Source: CAD feature listing. Evaluate the final solid. Frame: model axes, mm. Face numbers are marked on the shaded views. A direction names the side the tool comes from. Give positions to 0.01 mm unless a question says otherwise; leave off trailing zeros. Write each loop counter-clockwise with the first axis right and the second up, starting at its lowest first coordinate (ties: lowest second). Pieces come first, ordered by that corner, then holes.
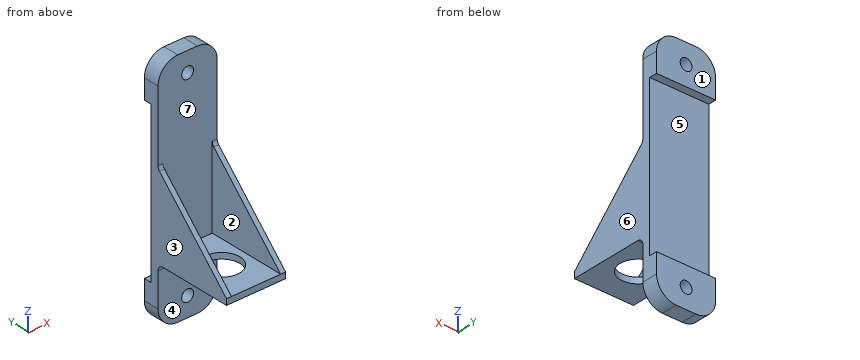
```python
from build123d import *

# Parameters (mm, degrees)
SKETCH1_W           = 30
SKETCH1_H           = 120
BOSS_EXTRUDE1_DEPTH = 8
SKETCH2_W           = 30
SKETCH2_H           = 80
CUT_EXTRUDE1_DEPTH  = 4
SKETCH3_W           = 30
SKETCH3_H           = 3
BOSS_EXTRUDE2_DEPTH = 40
SKETCH4_R           = 9.1
CUT_EXTRUDE2_DEPTH  = 40
BOSS_EXTRUDE3_DEPTH = 2.5
BOSS_EXTRUDE4_DEPTH = 2.5
SKETCH7_R           = 3
CUT_EXTRUDE3_DEPTH  = 131
FILLET1_R           = 10
FILLET2_R           = 3
FILLET3_R           = 3


with BuildPart() as part:
    # Sketch1 → Boss-Extrude1 (new body)
    with BuildSketch(Plane(origin=(0, 0, 0), x_dir=(1, 0, 0), z_dir=(0, 1, 0))):
        with Locations((15, 60)):
            Rectangle(SKETCH1_W, SKETCH1_H)
    extrude(amount=BOSS_EXTRUDE1_DEPTH)

    # Sketch2 → Cut-Extrude1 (cut)
    with BuildSketch(Plane(origin=(0, 8, 0), x_dir=(1, 0, 0), z_dir=(0, 1, 0))):
        with Locations((15, 60)):
            Rectangle(SKETCH2_W, SKETCH2_H)
    extrude(amount=-CUT_EXTRUDE1_DEPTH, mode=Mode.SUBTRACT)

    # Sketch3 → Boss-Extrude2 (add)
    with BuildSketch(Plane.XZ):
        with Locations((15, -88.5)):
            Rectangle(SKETCH3_W, SKETCH3_H)
    extrude(amount=BOSS_EXTRUDE2_DEPTH)

    # Sketch4 → Cut-Extrude2 (cut)
    with BuildSketch(Plane.XY.offset(-87)):
        with Locations((15, -20)):
            Circle(SKETCH4_R)
    extrude(amount=-CUT_EXTRUDE2_DEPTH, mode=Mode.SUBTRACT)

    # Sketch5 → Boss-Extrude3 (add)
    with BuildSketch(Plane(origin=(30, 0, 0), x_dir=(0, 0, -1), z_dir=(1, 0, 0))):
        Polygon((87, -40), (47, 0), (87, 0), align=None)
    extrude(amount=-BOSS_EXTRUDE3_DEPTH)

    # Sketch6 → Boss-Extrude4 (add)
    with BuildSketch(Plane.ZY):
        Polygon((-47, 0), (-87, -40), (-87, 0), align=None)
    extrude(amount=-BOSS_EXTRUDE4_DEPTH)

    # Sketch7 → Cut-Extrude3 (cut, through all)
    with BuildSketch(Plane(origin=(0, 0, 0), x_dir=(-1, 0, 0), z_dir=(0, -1, 0))):
        with Locations(Location((-15, 10, 0), (0, 0, 90))):
            Circle(SKETCH7_R)
        with Locations(Location((-15, 110, 0), (0, 0, 90))):
            Circle(SKETCH7_R)
    extrude(amount=-CUT_EXTRUDE3_DEPTH, mode=Mode.SUBTRACT)

    # Fillet1
    fillet1_edges = [part.edges().sort_by_distance(p)[0] for p in [
        (0, 4, -120),
        (30, 4, -120),
        (30, 4, 0),
        (0, 4, 0),
    ]]
    fillet(fillet1_edges, radius=FILLET1_R)

    # Fillet2
    fillet2_edges = [part.edges().sort_by_distance(p)[0] for p in [
        (15, 0, -90),
    ]]
    fillet(fillet2_edges, radius=FILLET2_R)

    # Fillet3
    fillet3_edges = [part.edges().sort_by_distance(p)[0] for p in [
        (28.75, 0, -47),
        (1.25, 0, -47),
    ]]
    fillet(fillet3_edges, radius=FILLET3_R)


solid = part.part
```
1. Access query for the marked faces 4, 5, 6 and 7. Directions: +Z, -Z, +X, -X, +Y, -Y. A direction counts if a zero-diameter tool reaches every point of the face in a straight line with its end or side. Return the directions, or none.
2. Section query C-C (z = -8.5). Return loops of the section in (x, y).
3. Pull-direction query (X, two-part tool) for the marked faces 1, 2 and 3; classes: pulls with the +X half, pulls with the -X half, needs draft (parallel to the pull), parting line crosses it, or undercut.
4. Section query D-D (y = -9.5). Return loops of the section in (x, z), plus the area to 4 significant figures.
5. Section query A-A (x = 15). Return loops of the section in (y, z), plus the area to 3 significant figures.
6. Pin query (flat end, axial travel): P1, Ø5, axis at x = 15, z = -10, coming from the +Y side; P2, Ø12.5, axis at x = 17, y = -29, coming from the +Z side; P3, Ø12, axis at x = 4, y = -17, coming from the -Z side; P4, Ø13.5, axis at x = 15, z = -111.5, coming from the -Y side. Return the tip coordinate at first contact, or that it passes through.
7. Section query B-B (y = -20). Return loops of the section in (x, z).
8. Line query: probe 1 along Y at (x, z) = (15, -88.3); probe 2 along Y at (x, z) = (11, -27); probe 3 along Y at (x, z) = (27.75, -107.5). Output: solid intervals per line, ascending.
The answers:
1. face 4: -Z, +X, -X, -Y
1. face 5: +X, -X, +Y
1. face 6: +Z, -Z, +X, +Y, -Y
1. face 7: +Z, -Y
2. outline: (0.11, 0) - (12.4, 0) - (12.4, 8) - (0.11, 8) - close; (17.6, 0) - (29.89, 0) - (29.89, 8) - (17.6, 8) - close
3. face 1: needs draft
3. face 2: undercut
3. face 3: pulls with the -X half
4. outline: (0, -90) - (30, -90) - (30, -56.5) - (27.5, -56.5) - (27.5, -87) - (2.5, -87) - (2.5, -56.5) - (0, -56.5) - close
4. area: 242.5 mm2
5. outline: (-40, -90) - (-29.1, -90) - (-29.1, -87) - (-40, -87) - close; (-10.9, -90) - (-3, -90) arc R3 cw to (0, -93) - (0, -107) - (8, -107) - (8, -100) - (4, -100) - (4, -20) - (8, -20) - (8, -13) - (0, -13) - (0, -87) - (-10.9, -87) - close; (0, -120) - (8, -120) - (8, -113) - (0, -113) - close; (0, -7) - (8, -7) - (8, 0) - (0, 0) - close
5. area: 611 mm2
6. P1: passes through
6. P2: stops at z = -87
6. P3: stops at z = -90
6. P4: stops at y = 0
7. outline: (0, -90) - (5.9, -90) - (5.9, -87) - (2.5, -87) - (2.5, -67) - (0, -67) - close; (24.1, -90) - (30, -90) - (30, -67) - (27.5, -67) - (27.5, -87) - (24.1, -87) - close
8. probe 1: y = -40 to -29.1, -10.9 to 4
8. probe 2: y = 0 to 4
8. probe 3: y = 0 to 8
